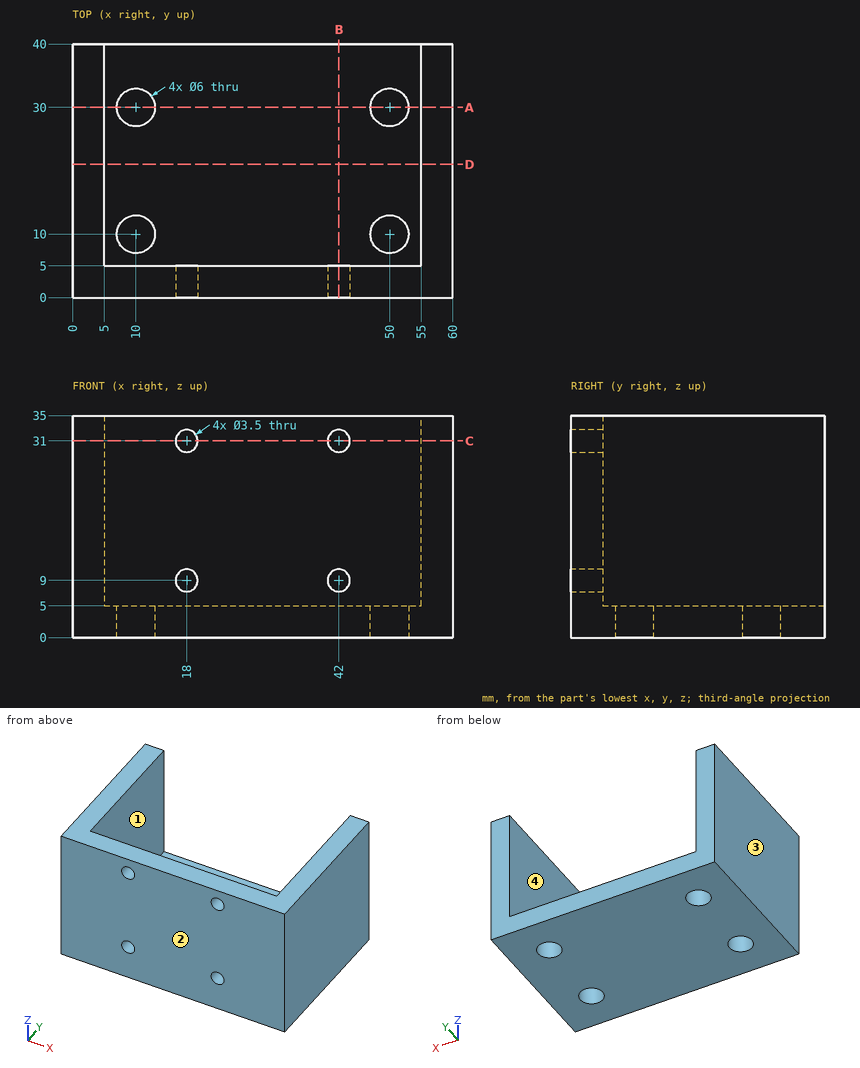
Geometry: see drawing. Coordinates: mm, zero at the bounding-box minimum. Give positions to 0.01 mm unless a question says otherwise; leave off trailing zeros. Write each loop counter-clockwise with the first axis right and the second up, starting at its lowest first coordinate (ties: lowest second). Pieces come first, ordered by that corner, then holes. Notation, with made-up numbers: M 82,36.25 L 111,36.25 A8 ccw 111,51.25 Z; hole C 65,13.25 d3. An arc over 180 degrees is marked long. Answer in a Markdown table with one row per item. Add a question column.
(1) Section A-A on y = 30. Return loops of the section in (x, z).
(2) Section D-D on y = 21. Return loops of the section in (x, z), and give its area (3 significant figures).
(3) First-contact query: pin 1 (5 mm diameter, centred on x = 50, y = 30, fed in from +Z); pin 2 (4 mm diameter, centred on x = 52, y = 22.5, fed in from +Z); pin 3 (9 mm diameter, centred on x = 19.5, z = 19.5, fed in from +Y). Flat tips, straight axial feed; report the tip coordinate or a pass-through.
(4) Mould query, pull axis X, two halves, no side actions, for the marked faces 1, 2, 3 and 4. Classes: +X half, -X half, draft (parallel to the pull), parting line (faces both ways), or undercut.
(5) Section C-C on z = 31. Return loops of the section in (x, y), and give its area (3 significant figures).
(6) Ray query, line 1 (Y direction, x = 10, z = 1); line 2 (X direction, y = 3, z = 9); line 3 (X direction, y = 7.5, z = 4). Return the intervals inside material, ascending.
(7) Section B-B on x = 42. Return loops of the section in (y, z).
Result set:
| question | item | result |
|---|---|---|
| 1 | outline | M 0,0 L 7,0 L 7,5 L 5,5 L 5,35 L 0,35 Z; M 13,0 L 47,0 L 47,5 L 13,5 Z; M 53,0 L 60,0 L 60,35 L 55,35 L 55,5 L 53,5 Z |
| 2 | outline | M 0,0 L 60,0 L 60,35 L 55,35 L 55,5 L 5,5 L 5,35 L 0,35 Z |
| 2 | area | 600 mm^2 |
| 3 | pin 1 | passes through |
| 3 | pin 2 | stops at z = 5 |
| 3 | pin 3 | stops at y = 5 |
| 4 | face 1 | undercut |
| 4 | face 2 | draft |
| 4 | face 3 | -X half |
| 4 | face 4 | undercut |
| 5 | outline | M 0,0 L 16.25,0 L 16.25,5 L 5,5 L 5,40 L 0,40 Z; M 19.75,0 L 40.25,0 L 40.25,5 L 19.75,5 Z; M 43.75,0 L 60,0 L 60,40 L 55,40 L 55,5 L 43.75,5 Z |
| 5 | area | 615 mm^2 |
| 6 | line 1 | y = 0 to 7, 13 to 27, 33 to 40 |
| 6 | line 2 | x = 0 to 16.25, 19.75 to 40.25, 43.75 to 60 |
| 6 | line 3 | x = 0 to 8.34, 11.66 to 48.34, 51.66 to 60 |
| 7 | outline | M 0,0 L 40,0 L 40,5 L 5,5 L 5,7.25 L 0,7.25 Z; M 0,10.75 L 5,10.75 L 5,29.25 L 0,29.25 Z; M 0,32.75 L 5,32.75 L 5,35 L 0,35 Z |
